```python
from build123d import *

# Parameters (mm, degrees)
SKETCH1_W           = 84
SKETCH1_H           = 38
BOSS_EXTRUDE1_DEPTH = 5
SKETCH2_W           = 84
SKETCH2_H           = 41.155299277
CUT_REVOLVE1_ANGLE  = 3
SKETCH3_R           = 6.3
SKETCH5_R           = 3.335164517
SKETCH3_4_R         = 6.3
SKETCH5_4_R         = 3.4
SKETCH5_8_R         = 3.335164517
SKETCH5_8_R_2       = 3.4
BOSS_EXTRUDE2_DEPTH = 3


with BuildPart() as part:
    # Sketch1 → Boss-Extrude1 (new body)
    with BuildSketch(Plane.XY):
        Rectangle(SKETCH1_W, SKETCH1_H)
    extrude(amount=BOSS_EXTRUDE1_DEPTH)

    # Sketch2 → Cut-Revolve1 (revolve, cut)
    with BuildSketch(Plane.XY.offset(5)):
        with Locations((0, 1.577649639)):
            Rectangle(SKETCH2_W, SKETCH2_H)
    revolve(axis=Axis((-42, -19, 5), (-1, 0, 0)), revolution_arc=CUT_REVOLVE1_ANGLE, mode=Mode.SUBTRACT)

    # Sketch3 → Loft2 section 0
    with BuildSketch(Plane(origin=(0, 0.209279164, 3.993284337), x_dir=(1, 0, 0), z_dir=(0, 0.052335956, 0.998629535))):
        with Locations((-29.895651858, 3.664359058)):
            Circle(SKETCH3_R)
    # Sketch5 → Loft2 section 1
    with BuildSketch(Plane(origin=(0, 0.361053437, 6.889309988), x_dir=(-1, 0, 0), z_dir=(0, -0.052335956, -0.998629535))):
        with Locations((29.895651858, 3.664359058)):
            Circle(SKETCH5_R)
    loft()

    # Sketch3<4> → Loft3 section 0
    with BuildSketch(Plane(origin=(0, 0.209279164, 3.993284337), x_dir=(1, 0, 0), z_dir=(0, 0.052335956, 0.998629535))):
        with Locations((29.895651858, 3.664359058)):
            Circle(SKETCH3_4_R)
    # Sketch5<4> → Loft3 section 1
    with BuildSketch(Plane(origin=(0, 0.361053437, 6.889309988), x_dir=(-1, 0, 0), z_dir=(0, -0.052335956, -0.998629535))):
        with Locations((-29.895651858, 3.664359058)):
            Circle(SKETCH5_4_R)
    loft()

    # Sketch5<8> → Boss-Extrude2 (add)
    with BuildSketch(Plane(origin=(0, 0.361053437, 6.889309988), x_dir=(-1, 0, 0), z_dir=(0, -0.052335956, -0.998629535))):
        with Locations((29.895651858, 3.664359058)):
            Circle(SKETCH5_8_R)
        with Locations((-29.895651858, 3.664359058)):
            Circle(SKETCH5_8_R_2)
    extrude(amount=-BOSS_EXTRUDE2_DEPTH)


solid = part.part
```
Build history of the part. All positions in model axes, mm. Coordinates: 2 decimals unless noted, no trailing zeros. Order: outer loops, then holes, each group sorted by start corner. A loop starts at its lowest first (then second) coordinate and runs counter-clockwise, first axis right, second up.
Item 1: Saw through at B-B on y = -10. List the corners of the cut face in (x, z), then the cut area to 3 significant figures.
Filled in:
outline: (-42, 0) - (42, 0) - (42, 4.53) - (-42, 4.53) - close
area: 380 mm2
Item 2: Drill centre lines: L1, parallel to X at y = 0, z = 4.25; L2, parallel to X at y = 1, z = 7.25; L3, parallel to Z at x = -32.5, y = 5. Where is each one in solid material? Low to high.
Filled in:
L1: x = -34.53 to -25.26, 25.25 to 34.54
L2: x = -31.26 to -28.54, 28.38 to 31.41
L3: z = 0 to 9.65
Item 3: Saw through at A-A on x = -22.5. List the corners of the cut face in (y, z), then the cut area to 3 significant figures.
Filled in:
outline: (-19, 0) - (19, 0) - (19, 3.01) - (-19, 5) - close
area: 152 mm2
Item 4: Drop flat-ended pins along their axis: pin 1 Ø2 at (y, z) = (-12, 5.5) entering from -X; pin 2 Ø1 at (x, y) = (-33, -10.5) entering from +Z; pin 3 Ø1 at (x, y) = (-26, 7.5) entering from +Z. Give the stop position or say it passes through.
Filled in:
pin 1: stops at x = -42
pin 2: stops at z = 4.58
pin 3: stops at z = 5.12
Item 5: Mould opens along Y. For faces 1 (the conical face through (-26.577, 5.057, 6.502)), 2 (the flat face through (-1, 19, 1)), 3 (the cylindrical face through (26.653, 5.118, 8.121)) say: released by +Y, released by -Y, zero draft, split by the parting line, or undercut.
Filled in:
face 1: undercut
face 2: released by +Y
face 3: split by the parting line
